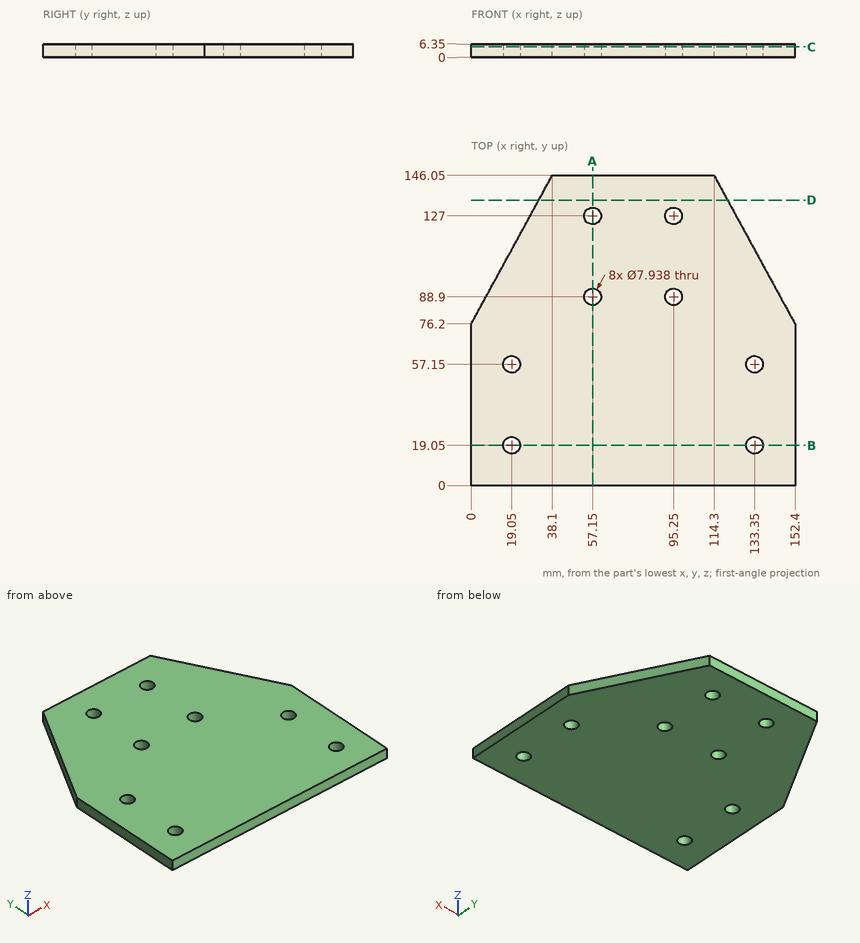
The figure shows three views and two pictorial views of one solid part (mm, origin at its lowest corner). Answer the questions. Round coordinates to 2 decimals unless told otherwise and drop trailing zeros. Loops run counter-clockwise (first coordinate to the right, second up) from the corner with the lowest first, then second, coordinate; pieces in that order, holes last. Notation, with made-up numbers: M 67,56.5 L 123,56.5 A15 ccw 123,71.5 Z; hole C -12,-31.5 d3. An arc over 180 degrees is marked long. Return JSON: item names as keys, results as strings.
Q1. Find section B-B, the plane y = 19.05. Determine the outline of the cut face in (x, z).
Results list:
{"outline": "M 0,0 L 15.08,0 L 15.08,6.35 L 0,6.35 Z; M 23.02,0 L 129.38,0 L 129.38,6.35 L 23.02,6.35 Z; M 137.32,0 L 152.4,0 L 152.4,6.35 L 137.32,6.35 Z"}
Q2. This flat-tipped pin is pushed along its axis until it touches: pin 1 Ø3 at (y, z) = (87.5, 1) entering from +X (1 decimal). Where does it stop, or does it pass through?
Results list:
{"pin 1": "stops at x = 147.1"}
Q3. Find the intervals of material crossed by line 1 along Y through (x, z) = (57.15, 4); line 2 along Y through (x, z) = (133.35, 4.25) (1 decimal); line 3 along X through (y, z) = (22, 1.75) (1 decimal), in increasing order. Write a range as from..to.
Results list:
{"line 1": "y = 0..84.93, 92.87..123.03, 130.97..146.05", "line 2": "y = 0..15.1, 23..53.2, 61.1..111.1", "line 3": "x = 0..16.4, 21.7..130.7, 136..152.4"}
Q4. Find section D-D, the plane y = 134.5. Determine the outline of the cut face in (x, z).
Results list:
{"outline": "M 31.8,0 L 120.6,0 L 120.6,6.35 L 31.8,6.35 Z"}
Q5. Find section A-A, the plane x = 57.15. Determine the outline of the cut face in (y, z).
Results list:
{"outline": "M 0,0 L 84.93,0 L 84.93,6.35 L 0,6.35 Z; M 92.87,0 L 123.03,0 L 123.03,6.35 L 92.87,6.35 Z; M 130.97,0 L 146.05,0 L 146.05,6.35 L 130.97,6.35 Z"}
Q6. Find section C-C, the plane z = 5. State how many separate pieces and enclosed holes the cut face has, plus the area to 3 significant figures.
Results list:
{"separate pieces": "1", "enclosed holes": "8", "area": "19,200 mm2"}
